For this review, take the finished solid that the model builds, in its own axes (mm). A direction names the side the tool comes from. Coordinates: 2 decimals unless noted, no trailing zeros. Loops run counter-clockwise (first coordinate to the right, second up) from the corner with the lowest first, then second, coordinate; pieces in that order, holes last. Notation, with made-up numbers: M 65.25,19 L 120.25,19 A20 cw 120.25,32 Z; hole C 41,-39 d3. An arc over 180 degrees is marked long. Put each result on its own line as item: value.
```python
from build123d import *
from build123d.topology import SkipClean

# Parameters (mm, degrees)
BOSS_EXTRUDE1_DEPTH     = 4
SKETCH3_W               = 5
SKETCH3_H               = 30
BOSS_EXTRUDE3_DEPTH     = 24
BOSS_EXTRUDE5_DEPTH     = 5
SKETCH7_3_R             = 3.25755
CUT_EXTRUDE3_DEPTH      = 5
FILLET3_R               = 10
CUT_EXTRUDE4_DEPTH      = 25
CUT_EXTRUDE4_DEPTH_BACK = 1
CUT_EXTRUDE5_DEPTH      = 50.494221145
CUT_EXTRUDE5_DEPTH_BACK = 50.494221145
SKETCH9_R               = 2.75
FILLET4_R               = 1
FILLET5_R               = 3
BOSS_EXTRUDE6_DEPTH     = 4
FILLET6_R               = 2
BOSS_EXTRUDE7_DEPTH     = 4


with BuildPart() as part:
    # Sketch2 → Boss-Extrude1 (new body)
    with BuildSketch(Plane(origin=(0, 0, 0), x_dir=(1, 0, 0), z_dir=(0, 1, 0))):
        with BuildLine():
            Line((18.000912404, -14.946929254), (18.000912404, 15.053070746))
            Line((18.000912404, 15.053070746), (0.039090451, 15.053070746))
            ThreePointArc((0.039090451, 15.053070746), (-10.199781301, 11.024824414), (-14.94907539, 1.099832277))
            Line((-14.94907539, 1.099832277), (-5.983249792, 0.448020006))
            ThreePointArc((-5.983249792, 0.448020006), (3.000957071, 5.20912276), (3.369824569, -4.951979994))
            Line((3.369824569, -4.951979994), (10.151696986, -14.946929254))
            Line((10.151696986, -14.946929254), (18.000912404, -14.946929254))
        make_face()
    boss_extrude1 = extrude(amount=BOSS_EXTRUDE1_DEPTH)

    # Sketch3 → Boss-Extrude3 (add)
    with BuildSketch(Plane(origin=(0, 4, 0), x_dir=(1, 0, 0), z_dir=(0, 1, 0))):
        with Locations((15.500912404, 0.053070746)):
            Rectangle(SKETCH3_W, SKETCH3_H)
    extrude(amount=BOSS_EXTRUDE3_DEPTH)

    # Mirror1: Boss-Extrude1 across plane
    add(boss_extrude1.mirror(Plane.ZX.offset(16)))

    # Sketch7 → Boss-Extrude5 (add)
    with BuildSketch(Plane.ZY.offset(-13.000912404)):
        with BuildLine():
            Line((-15.053070746, 0), (-15.053070746, 4))
            Line((-15.053070746, 4), (-15.053070746, 7.075913265))
            ThreePointArc((-15.053070746, 7.075913265), (-18.310620746, 10.333463265), (-15.053070746, 13.591013265))
            Line((-15.053070746, 13.591013265), (-15.053070746, 20.666926531))
            ThreePointArc((-15.053070746, 20.666926531), (-25.386534011, 10.333463265), (-15.053070746, 0))
        make_face()
        with BuildLine():
            ThreePointArc((25.146929254, 21.8), (22.159418422, 29.012489168), (14.946929254, 32))
            Line((14.946929254, 32), (14.946929254, 28))
            Line((14.946929254, 28), (14.946929254, 25.05755))
            ThreePointArc((14.946929254, 25.05755), (17.250364949, 24.103435695), (18.204479254, 21.8))
            ThreePointArc((18.204479254, 21.8), (17.250364949, 19.496564305), (14.946929254, 18.54245))
            Line((14.946929254, 18.54245), (14.946929254, 11.6))
            ThreePointArc((14.946929254, 11.6), (22.159418422, 14.587510832), (25.146929254, 21.8))
        make_face()
        with BuildLine():
            Line((14.946929254, 28), (14.946929254, 32))
            ThreePointArc((14.946929254, 32), (4.746929254, 21.8), (14.946929254, 11.6))
            Line((14.946929254, 11.6), (14.946929254, 18.54245))
            ThreePointArc((14.946929254, 18.54245), (11.689379254, 21.8), (14.946929254, 25.05755))
            Line((14.946929254, 25.05755), (14.946929254, 28))
        make_face()
    extrude(amount=-BOSS_EXTRUDE5_DEPTH)

    # Sketch7<3> → Cut-Extrude3 (cut)
    with SkipClean():  # the faces are left unmerged after this step: merging them gives an invalid solid
        with BuildSketch(Plane.ZY.offset(-13.000912404)):
            with Locations((14.946929254, 21.8)):
                Circle(SKETCH7_3_R)
            with Locations((-15.053070746, 10.333463265)):
                Circle(SKETCH7_3_R)
        extrude(amount=-CUT_EXTRUDE3_DEPTH, mode=Mode.SUBTRACT)

    # Fillet3
    # the kernel refuses this fillet: 10 mm, written as the material it adds along each edge
    with BuildSketch(Plane(origin=(13.000912404, 20.666926531, -15.053070746), x_dir=(0, -0.25425566101904284, -0.9671370424297528), z_dir=(1, 0, 0))) as fillet3_piece_1:
        with BuildLine():
            CenterArc((7.797239676, 9.671370424), FILLET3_R, 194.729484057, 60.541031886)
            Line((-1.874130748, 7.128813814), (0, 0))
            ThreePointArc((0, 0), (2.627341533, 0.339588165), (5.254683066, 0))
        make_face()
    extrude(amount=5)
    with BuildSketch(Plane(origin=(13.000912404, 11.6, 14.946929254), x_dir=(0, -1, 0), z_dir=(1, 0, 0))) as fillet3_piece_2:
        with BuildLine():
            CenterArc((7.351068344, -10), FILLET3_R, 90, 60.326985198)
            ThreePointArc((-1.337579351, -5.04950495), (-0.340063626, -2.611829759), (0, 0))
            Line((0, 0), (7.351068344, 0))
        make_face()
    extrude(amount=5)

    # Sketch8 → Cut-Extrude4 (cut, two sides: drawn at the far end of the back side and taken through both)
    with SkipClean():  # the faces are left unmerged after this step: merging them gives an invalid solid
        with BuildSketch(Plane(origin=(0, 4, 0), x_dir=(1, 0, 0), z_dir=(0, 1, 0)).offset(-CUT_EXTRUDE4_DEPTH_BACK)):
            with BuildLine():
                Line((-7.47930432, 0.556782628), (-5.983249792, 0.448020006))
                ThreePointArc((-5.983249792, 0.448020006), (3.000957071, 5.20912276), (3.369824569, -4.951979994))
                Line((3.369824569, -4.951979994), (4.217763535, -6.201650648))
                ThreePointArc((4.217763535, -6.201650648), (5.494951676, -5.104459431), (6.495190528, -3.75))
                ThreePointArc((6.495190528, -3.75), (7.244443697, -1.941142838), (7.5, 0))
                ThreePointArc((7.5, 0), (1.941142838, 7.244443697), (-6.495190528, 3.75))
                ThreePointArc((-6.495190528, 3.75), (-7.167341617, 2.208894325), (-7.47930432, 0.556782628))
            make_face()
            with BuildLine():
                Line((-8.304173093, 0.616750289), (-7.47930432, 0.556782628))
                ThreePointArc((-7.47930432, 0.556782628), (-7.167341617, 2.208894325), (-6.495190528, 3.75))
                Line((-6.495190528, 3.75), (-8.304173093, 0.616750289))
            make_face()
            with BuildLine():
                ThreePointArc((4.217763535, -6.201650648), (-3.752135014, -6.49395741), (-7.47930432, 0.556782628))
                Line((-7.47930432, 0.556782628), (-8.304173093, 0.616750289))
                Line((-8.304173093, 0.616750289), (-11.199802547, -4.398627047))
                Line((-11.199802547, -4.398627047), (1.534433746, -12.342282792))
                Line((1.534433746, -12.342282792), (4.683468483, -6.887994631))
                Line((4.683468483, -6.887994631), (4.217763535, -6.201650648))
            make_face()
            with BuildLine():
                ThreePointArc((6.495190528, -3.75), (5.494951676, -5.104459431), (4.217763535, -6.201650648))
                Line((4.217763535, -6.201650648), (4.683468483, -6.887994631))
                Line((4.683468483, -6.887994631), (6.495190528, -3.75))
            make_face()
            with BuildLine():
                Line((3.369824569, -4.951979994), (-5.983249792, 0.448020006))
                Line((-5.983249792, 0.448020006), (-7.47930432, 0.556782628))
                ThreePointArc((-7.47930432, 0.556782628), (-3.752135014, -6.49395741), (4.217763535, -6.201650648))
                Line((4.217763535, -6.201650648), (3.369824569, -4.951979994))
            make_face()
        extrude(amount=CUT_EXTRUDE4_DEPTH + CUT_EXTRUDE4_DEPTH_BACK, mode=Mode.SUBTRACT)

    # Sketch9 → Cut-Extrude5 (cut, two sides: drawn at the far end of the back side and taken through both)
    with BuildSketch(Plane.ZY.offset(-13.000912404).offset(-CUT_EXTRUDE5_DEPTH_BACK)):
        with Locations((9, 10.2)):
            Circle(SKETCH9_R)
        with Locations((-9, 21.8)):
            Circle(SKETCH9_R)
    extrude(amount=CUT_EXTRUDE5_DEPTH + CUT_EXTRUDE5_DEPTH_BACK, mode=Mode.SUBTRACT)

    # Fillet4
    fillet4_edges = [part.edges().sort_by_distance(p)[0] for p in [
        (13.000912404, 4, -0.053070746),
        (13.000912404, 28, -0.053070746),
    ]]
    fillet(fillet4_edges, radius=FILLET4_R)

    # Fillet5
    fillet5_edges = [part.edges().sort_by_distance(p)[0] for p in [
        (10.151696986, 2, 14.946929254),
        (-14.94907539, 2, -1.099832277),
        (10.151696986, 30, 14.946929254),
        (-14.94907539, 30, -1.099832277),
    ]]
    fillet(fillet5_edges, radius=FILLET5_R)

    # Sketch10 → Boss-Extrude6 (add)
    with BuildSketch(Plane.XZ):
        with BuildLine():
            ThreePointArc((0.039090451, -15.053070746), (-5.733491903, -13.900038334), (-10.620178824, -10.617892431))
            Line((-10.620178824, -10.617892431), (-9.005905934, -15.053070746))
            Line((-9.005905934, -15.053070746), (0.039090451, -15.053070746))
        make_face()
    extrude(amount=-BOSS_EXTRUDE6_DEPTH)

    # Fillet6
    fillet6_edges = [part.edges().sort_by_distance(p)[0] for p in [
        (-9.005905934, 2, -15.053070746),
    ]]
    fillet(fillet6_edges, radius=FILLET6_R)

    # Sketch11 → Boss-Extrude7 (add)
    with BuildSketch(Plane(origin=(0, 32, 0), x_dir=(1, 0, 0), z_dir=(0, 1, 0))):
        with BuildLine():
            Line((-9.484876099, 13.737111032), (-10.620178824, 10.617892431))
            ThreePointArc((-10.620178824, 10.617892431), (-5.733491903, 13.900038334), (0.039090451, 15.053070746))
            Line((0.039090451, 15.053070746), (-7.605490857, 15.053070746))
            ThreePointArc((-7.605490857, 15.053070746), (-8.75264373, 14.691374834), (-9.484876099, 13.737111032))
        make_face()
    extrude(amount=-BOSS_EXTRUDE7_DEPTH)


solid = part.part
```
(1) Draft analysis for pull direction Y (two halves, no side actions). For faces 1 (the flat face through (5, 0, -7)), 2 (the flat face through (-10.045, 30.028, -12.199)), 3 (the flat face through (5.6, 28.5, 5.3)), state which applies: +Y half, -Y half, draft (parallel to the pull), parting line (faces both ways), or undercut.
Determined:
face 1: -Y half
face 2: draft
face 3: undercut
(2) Add section D-D (y = 17). Write out the cut boundary in (x, z), plus the area to 3 significant figures.
Determined:
outline: M 13,-22.95 L 18,-22.95 L 18,23.95 L 13,23.95 Z
area: 234 mm^2
(3) Tool access review of faces 4 (the flat face through (3, 2, -15.053)), 5 (the flat face through (12, 30, 14.947)), 6 (the flat face through (-7.387, 28.493, -2.205)), 7 (the flat face through (4, 4, -7)), 8 (the flat face through (5, 30, -15.053)): name each direction out of +Z, -Z, +X, -X, +Y, -Y from which nothing blocks a thin tool from reaching the whole face with its end or side.
Determined:
face 4: -Z, -X, +Y, -Y
face 5: +Z, -X, +Y, -Y
face 6: +Z
face 7: +Z, -Z, -X
face 8: -Z, +X, -X, +Y
(4) Add section C-C (z = -9). Write out the cut boundary in (x, y).
Determined:
outline: M -12.01,0 L 18,0 L 18,19.05 L 13,19.05 L 13,5 A1 cw 12,4 L -12.01,4 Z; M -12.01,28 L 12,28 A1 cw 13,27 L 13,24.55 L 18,24.55 L 18,32 L -12.01,32 Z
(5) Wall thickness on line 1 along Y through (x, z) = (10.5, -6.5); line 2 along Z through (x, y) = (14, 21); line 3 along Y through (x, z) = (15.25, -9): over which ranges is each line inside the solid? List them lowest first. Write a range as [from, to].
Determined:
line 1: y = [0, 4], [28, 32]
line 2: z = [-17.95, -11.63], [-6.37, 11.79], [18.1, 25.12]
line 3: y = [0, 19.05], [24.55, 32]
(6) Add section B-B (z = 2.5). Write out the cut boundary in (x, y), plus the area to 3 significant figures.
Determined:
outline: M 5.45,0 L 18,0 L 18,32 L 5.45,32 L 5.45,29 L 7.07,29 L 7.07,28 L 12,28 A1 cw 13,27 L 13,5 A1 cw 12,4 L 7.07,4 L 7.07,3 L 5.45,3 Z
area: 218 mm^2
(7) Add section A-A (z = 9.5). Write out the cut boundary in (x, y).
Determined:
outline: M 6.46,0 L 18,0 L 18,7.5 L 13,7.5 L 13,5 A1 cw 12,4 L 6.46,4 Z; M 6.46,28 L 12,28 A1 cw 13,27 L 13,12.9 L 18,12.9 L 18,32 L 6.46,32 Z
(8) For pin 1 (9 mm diameter, centred on y = 10.2, z = 9, fed in from -X); pin 2 (4 mm diameter, centred on y = 10.33, z = -15.05, fed in from +X); pin 3 (5 mm diameter, centred on x = 14.5, y = 26.5, fed in from -Z); pin 4 (3.5 mm diameter, centred on x = 13.5, y = 1, fed in from +Z), all flat-tipped, find the tip position at first contact; note any pin that passes through.
Determined:
pin 1: stops at x = 13
pin 2: passes through
pin 3: stops at z = -15.9
pin 4: stops at z = 14.95
